from build123d import *

# Parameters (mm, degrees)
F0_W     = 76.2
F0_H     = 152.4
F0_R     = 6.35
F1_DEPTH = 25.4
F2_R     = 2.54
F3_R     = 6.35
F4_DEPTH = 12.7
F5_W     = 76.2
F5_H     = 12.7
F6_DEPTH = 12.7


with BuildPart() as f1:
    # F0 (on Front) → F1 (new body)
    with BuildSketch(Plane.XZ):
        Rectangle(F0_W, F0_H)
        with Locations((-25.4, -57.15)):
            Circle(F0_R, mode=Mode.SUBTRACT)
        with Locations((25.4, -57.15)):
            Circle(F0_R, mode=Mode.SUBTRACT)
        with Locations((-25.4, 57.15)):
            Circle(F0_R, mode=Mode.SUBTRACT)
        with Locations((25.4, 57.15)):
            Circle(F0_R, mode=Mode.SUBTRACT)
    extrude(amount=F1_DEPTH)

    # F2
    f2_edges = [f1.edges().sort_by_distance(p)[0] for p in [
        (-38.1, -12.7, 76.2),
        (-38.1, -12.7, -76.2),
        (38.1, -12.7, -76.2),
        (38.1, -12.7, 76.2),
    ]]
    fillet(f2_edges, radius=F2_R)

    # F3 (on face) → F4 (join)
    with BuildSketch(Plane.XZ.offset(25.4)):
        with BuildLine():
            ThreePointArc((38.1, 73.66), (37.3560512242, 75.4560512242), (35.56, 76.2))
            Line((35.56, 76.2), (-35.56, 76.2))
            ThreePointArc((-35.56, 76.2), (-37.3560512242, 75.4560512242), (-38.1, 73.66))
            Line((-38.1, 73.66), (-38.1, 38.1))
            Line((-38.1, 38.1), (38.1, 38.1))
            Line((38.1, 38.1), (38.1, 73.66))
        make_face()
        with Locations((-25.4, 57.15)):
            Circle(F3_R, mode=Mode.SUBTRACT)
        with Locations((25.4, 57.15)):
            Circle(F3_R, mode=Mode.SUBTRACT)
    extrude(amount=F4_DEPTH)

    # F5 (on face) → F6 (join)
    with BuildSketch(Plane(origin=(0, 0, 38.1), x_dir=(1, 0, 0), z_dir=(0, 0, -1))):
        with BuildLine():
            Line((-12.7, 82.0940905122), (-38.1, 38.1))
            Line((-38.1, 38.1), (38.1, 38.1))
            Line((38.1, 38.1), (12.7, 82.0940905122))
            ThreePointArc((12.7, 82.0940905122), (0, 69.3940905122), (-12.7, 82.0940905122))
        make_face()
        with BuildLine():
            Line((-6.35, 82.0940905122), (-12.7, 82.0940905122))
            ThreePointArc((-12.7, 82.0940905122), (0, 69.3940905122), (12.7, 82.0940905122))
            Line((12.7, 82.0940905122), (6.35, 82.0940905122))
            ThreePointArc((6.35, 82.0940905122), (0, 75.7440905122), (-6.35, 82.0940905122))
        make_face()
        with BuildLine():
            ThreePointArc((12.7, 82.0940905122), (0, 94.7940905122), (-12.7, 82.0940905122))
            Line((-12.7, 82.0940905122), (-6.35, 82.0940905122))
            ThreePointArc((-6.35, 82.0940905122), (0, 88.4440905122), (6.35, 82.0940905122))
            Line((6.35, 82.0940905122), (12.7, 82.0940905122))
        make_face()
        with Locations((0, 31.75)):
            Rectangle(F5_W, F5_H)
    extrude(amount=F6_DEPTH)

    # F7: F1 across plane


with BuildPart() as f1_1:
    add(f1.part)
    add(f1.part.mirror(Plane.XY))


solid = f1_1.part
The listing builds one solid part. Answer for the finished solid, in the listing's coordinates (mm). A direction names the side the tool comes from. Give positions to 0.01 mm unless a question says otherwise; leave off trailing zeros. Write each loop counter-clockwise with the first axis right and the second up, starting at its lowest first coordinate (ties: lowest second). Pieces come first, ordered by that corner, then holes.
1) For a pull along Z with two mould halves and no side action, classify faces 1 (the face through (-1, -53, 25.4)), 2 (the face through (25.578, -59.789, -31.839)), 3 (the face through (0, -19, 76.2)), 4 (the face through (-1, -25.4, 0)) as pulls with the +Z half, pulls with the -Z half, needs draft (parallel to the pull), parting line crosses it, or undercut.
2) Given P1, Ø6, axis at x = -2.5, y = -77, coming from the -Z side; P2, Ø14.5, axis at x = 0, y = -82.09, coming from the +Z side; P3, Ø14.5, axis at x = -25.4, z = 57.15, coming from the +Y side; P4, Ø11.5, axis at x = 0.5, z = -51.5, coming from the -Y side, each flat-ended and moving along its own axis, determine where each tip first touches the part or whether it passes through.
3) Section A-A (y = -29.5) is taken. Write down the section's boundary in (x, z), and give its area (3 significant figures).
4) Find the intervals of material crossed by L1, parallel to X at y = -21, z = -57.15; L2, parallel to Z at x = -25.4, y = -29; L3, parallel to Z at x = -0.5, y = -51, in increasing order.
5) Section C-C (x = 0) is taken. Write down the section's boundary in (y, z), and give its area (3 significant figures).
6) A tool of negligible diameter and unlimited length cuts with its end or side. For faces 5 (the face through (-1, -61, -38.1)), 6 (the face through (-1, -53, -25.4)), 7 (the face through (-1, -38.1, 57)), from which of +Z, -Z, +X, -X, +Y, -Y can it reach the whole face along a straight path? Write none if from no direction.
7) Section D-D (y = -40) is taken. Write down the section's boundary in (x, z).
8) Section B-B (z = -57.15) is taken. Write down the section's boundary in (x, y).
Response:
1. face 1: undercut
1. face 2: needs draft
1. face 3: pulls with the +Z half
1. face 4: undercut
2. P1: stops at z = -38.1
2. P2: stops at z = 38.1
2. P3: stops at y = 0
2. P4: stops at y = -38.1
3. outline: (-38.1, -73.66) arc R2.54 ccw to (-35.56, -76.2) - (35.56, -76.2) arc R2.54 ccw to (38.1, -73.66) - (38.1, -25.4) - (-38.1, -25.4) - close; (-38.1, 25.4) - (38.1, 25.4) - (38.1, 73.66) arc R2.54 ccw to (35.56, 76.2) - (-35.56, 76.2) arc R2.54 ccw to (-38.1, 73.66) - close; hole circle Ø12.7 at (-25.4, -57.15); hole circle Ø12.7 at (-25.4, 57.15); hole circle Ø12.7 at (25.4, -57.15); hole circle Ø12.7 at (25.4, 57.15)
3. area: 7,230 mm2
4. L1: x = -38.1 to -31.75, -19.05 to 19.05, 31.75 to 38.1
4. L2: z = -76.2 to -63.5, -50.8 to -25.4, 25.4 to 50.8, 63.5 to 76.2
4. L3: z = -38.1 to -25.4, 25.4 to 38.1
5. outline: (-94.79, -38.1) - (-88.44, -38.1) - (-88.44, -25.4) - (-94.79, -25.4) - close; (-94.79, 25.4) - (-88.44, 25.4) - (-88.44, 38.1) - (-94.79, 38.1) - close; (-75.74, -38.1) - (-38.1, -38.1) - (-38.1, -76.2) - (0, -76.2) - (0, 76.2) - (-38.1, 76.2) - (-38.1, 38.1) - (-75.74, 38.1) - (-75.74, 25.4) - (-25.4, 25.4) - (-25.4, -25.4) - (-75.74, -25.4) - close
5. area: 6,280 mm2
6. face 5: -Z, +X, -X, -Y
6. face 6: +X, -X, -Y
6. face 7: +Z, +X, -X, -Y
7. outline: (-37, -38.1) - (37, -38.1) - (37, -25.4) - (-37, -25.4) - close; (-37, 25.4) - (37, 25.4) - (37, 38.1) - (-37, 38.1) - close
8. outline: (-38.1, -38.1) - (-31.75, -38.1) - (-31.75, 0) - (-38.1, 0) - close; (-19.05, -38.1) - (19.05, -38.1) - (19.05, 0) - (-19.05, 0) - close; (31.75, -38.1) - (38.1, -38.1) - (38.1, 0) - (31.75, 0) - close
